Design review of the part built by this model. Coordinates are the model's own, in mm. Face numbers are marked on the shaded views. A direction names the side the tool comes from. Coordinates: 2 decimals unless noted, no trailing zeros. Loops run counter-clockwise (first coordinate to the right, second up) from the corner with the lowest first, then second, coordinate; pieces in that order, holes last. Notation, with made-up numbers: M 71.5,-5 L 119.5,-5 A15 ccw 119.5,3 Z; hole C 64,36.25 d1. An arc over 180 degrees is marked long. Answer as a JSON object with one key per item and string values. Group by question number.
1. Consider section D-D (z = 5.75). State the section outline as (x, y) points, then the cut area to 3 significant figures.
2. Insertion check: pin 1 (1.5 mm diameter, centred on x = 15.25, z = 4, fed in from -Y); pin 2 (2.5 mm diameter, centred on x = 7.5, z = 5.5, fed in from -Y); pin 3 (1.1 mm diameter, centred on y = 1, z = 2, fed in from +X); pin 4 (1.5 mm diameter, centred on y = 6, z = 7, fed in from +X). Each pin has a flat end and moves straight along its axis. Give the tip position at first contact, or say it passes through.
3. Machinability: for the marked faces 1 and 2, which of the approach directions +Z, -Z, +X, -X, +Y, -Y give a long, thin tool a straight path to every point of the face, cutting with its end or side? Answer none if there is none.
4. Consider section A-A (z = 3.75). State the section outline as (x, y) points, then the cut area to 3 significant figures.
5. Draft analysis for pull direction Z (two halves, no side actions). For the marked faces 3, 4 and 5, state which applies: +Z half, -Z half, draft (parallel to the pull), parting line (faces both ways), or undercut.
6. Consider section B-B (x = -3.25). State the section outline as (y, z) points.
7. Consider section C-C (y = 4.75). State the section outline as (x, z) points.
8. To check wall thickness, follow probe 1 along Y at (x, z) = (5.5, 1.75); probe 2 along X at (y, z) = (0.5, 7.25); probe 3 along Z at (x, y) = (-3.25, 4.75). State the ranges of each line that lie inside material, in increasing order.
Autodesk Fusion 360 part; units mm, degrees
sketch "Sketch1" plane through (0, 0, 0) normal (0, 1, 0) x (1, 0, 0) in component "CableClamp"
  line L0 (0, 0) -> (12, 0)
  line L1 (12, 0) -> (12, -8) construction
  line L2 (12, -8) -> (0, -8)
  line L3 (0, -8) -> (0, 0) construction
  circle A0 centre (15.25, -4) radius 1.25
  circle A1 centre (15.25, -4) radius 2.25
  line L4 (12, -4) -> (13, -4) construction
  line L5 (12, 0) -> (16.2016, -1.9612)
  line L6 (12, -8) -> (16.2016, -6.0388)
  circle A2 centre (-3.25, -4) radius 1.25
  circle A3 centre (-3.25, -4) radius 2.25
  line L7 (0, -4) -> (-1, -4) construction
  line L8 (0, -8) -> (-4.2016, -6.0388)
  line L9 (0, 0) -> (-4.2016, -1.9612)
  dimension "d5" = 12
  dimension "d6" = 8
  dimension "d7" = 2.5
  dimension "d10" = 1
  dimension "d11" = 1
  dimension "d12" = 2.5
  dimension "d13" = 1
  dimension "d14" = 1
extrude "Extrude1" add sketch "Sketch1" along normal blind 8 in component "CableClamp"
fillet "Fillet1" radius 7.25 4 edges at (0, 4, 0) (12, 4, 0) (12, 4, 8) (0, 4, 8) in component "CableClamp"
sketch "Sketch1 (1)" plane through (0, 0, 8) normal (0, 0, 1) x (1, 0, 0) in component "CableClamp"
  line L0 (1.6087, 8) -> (1.6087, 0)
  line L1 (1.6087, 0) -> (10.3913, 0)
  line L2 (10.3913, 0) -> (10.3913, 8)
  line L3 (10.3913, 8) -> (1.6087, 8)
  line L4 (1.6087, 2.38) -> (10.3913, 2.38)
  dimension "d31" = 2.38
extrude "Extrude2" cut sketch "Sketch1 (1)" against normal through all contours L0 L1 L2 L4 in component "CableClamp"
fillet "Fillet1'" radius 0.5 4 edges at (1.6087, 2.38, 4) (1.6087, 0, 4) (10.3913, 0, 4) (10.3913, 2.38, 4) in component "CableClamp"
component "CableClamp" placed x (1, 0, 0) y (0, 1, 0) z (0, 0, 1) at (0, 0, 0)
equation "width = 12 mm"
equation "height = 8 mm"
equation "screwHoleDiamerter = 2.5 mm"
equation "screwHoleWallThickness = 1 mm"
equation "d5 = width"
equation "d6 = height"
equation "d7 = screwHoleDiamerter"
equation "d10 = screwHoleWallThickness"
equation "d12 = screwHoleDiamerter"
equation "d13 = screwHoleWallThickness"
equation "thickness = 8 mm"
equation "d16 = thickness"
equation "cableDiameter = 3.4 mm"
equation "d31 = cableDiameter * clampRatio"
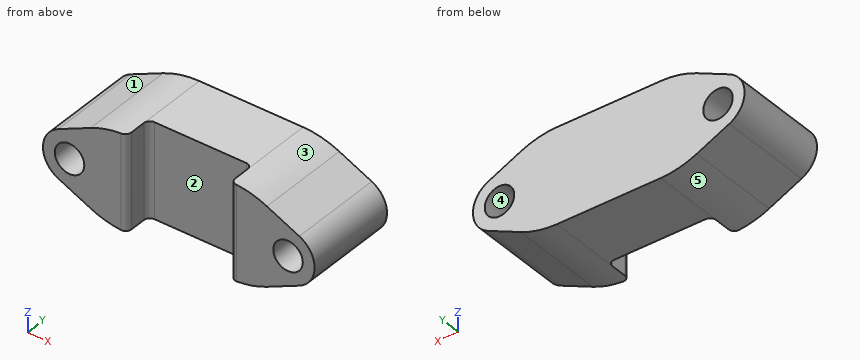
Findings below:
{
 "1": {"outline": "M -4.66,0 L 1.11,0 A0.5 ccw 1.61,0.5 L 1.61,1.88 A0.5 cw 2.11,2.38 L 9.89,2.38 A0.5 cw 10.39,1.88 L 10.39,0.5 A0.5 ccw 10.89,0 L 16.66,0 L 16.66,8 L -4.66,8 Z", "area": "150 mm^2"},
 "2": {"pin 1": "passes through", "pin 2": "stops at y = 2.38", "pin 3": "stops at x = 16.97", "pin 4": "stops at x = 15.75"},
 "3": {"face 1": "+Z, -X, +Y, -Y", "face 2": "+Z, -Z, -Y"},
 "4": {"outline": "M -5.49,0 L -4.47,0 L -4.47,8 L -5.49,8 Z; M -2.03,0 L 1.11,0 A0.5 ccw 1.61,0.5 L 1.61,1.88 A0.5 cw 2.11,2.38 L 9.89,2.38 A0.5 cw 10.39,1.88 L 10.39,0.5 A0.5 ccw 10.89,0 L 14.03,0 L 14.03,8 L -2.03,8 Z; M 16.47,0 L 17.49,0 L 17.49,8 L 16.47,8 Z", "area": "124 mm^2"},
 "5": {"face 3": "+Z half", "face 4": "undercut", "face 5": "-Z half"},
 "6": {"outline": "M 0,1.52 L 8,1.52 L 8,2.75 L 0,2.75 Z; M 0,5.25 L 8,5.25 L 8,6.48 L 0,6.48 Z"},
 "7": {"outline": "M -4.2,1.96 L -1.46,0.68 A7.25 ccw 1.61,0 L 10.39,0 A7.25 ccw 13.46,0.68 L 16.2,1.96 A2.25 ccw 16.2,6.04 L 13.46,7.32 A7.25 ccw 10.39,8 L 1.61,8 A7.25 ccw -1.46,7.32 L -4.2,6.04 A2.25 ccw Z; hole C -3.25,4 d2.5; hole C 15.25,4 d2.5"},
 "8": {"probe 1": "y = 2.38 to 8", "probe 2": "x = -1.61 to 1.61, 10.39 to 13.61", "probe 3": "z = 1.52 to 2.75, 5.25 to 6.48"}
}
